```python
from build123d import *

# Parameters (mm, degrees)
SKETCH_1_W          = 51
SKETCH_1_H          = 39
EXTRUDE_1_DEPTH     = 240
SKETCH_2_W          = 41.961119827
SKETCH_2_H          = 6.971123129
EXTRUDE_2_DEPTH     = 35
SKETCH_3_W          = 16.244799638
SKETCH_3_H          = 3.419957818
EXTRUDE_3_DEPTH     = 30
SKETCH_4_W          = 51
SKETCH_4_H          = 4.841751688
EXTRUDE_4_DEPTH     = 10
SKETCH_5_W          = 44.706396848
SKETCH_5_H          = 29.024048215
CUT_EXTRUDE_1_DEPTH = 10
SKETCH_6_W          = 34.715500368
SKETCH_6_H          = 26.036625276
CUT_EXTRUDE_2_DEPTH = 10


with BuildPart() as part:
    # 草图1 → 凸台-拉伸1 (new body)
    with BuildSketch(Plane(origin=(0, 0, 0), x_dir=(1, 0, 0), z_dir=(0, 1, 0))):
        with Locations((25.5, 19.5)):
            Rectangle(SKETCH_1_W, SKETCH_1_H)
    extrude(amount=EXTRUDE_1_DEPTH)

    # 草图2 → 凸台-拉伸2 (add)
    with BuildSketch(Plane(origin=(0, 240, 0), x_dir=(1, 0, 0), z_dir=(0, 1, 0))):
        with Locations((25.724627293, 35.514438435)):
            Rectangle(SKETCH_2_W, SKETCH_2_H)
    extrude(amount=EXTRUDE_2_DEPTH)

    # 草图3 → 凸台-拉伸3 (add)
    with BuildSketch(Plane(origin=(0, 240, 0), x_dir=(1, 0, 0), z_dir=(0, 1, 0))):
        with Locations((21.054054836, 2.926937994)):
            Rectangle(SKETCH_3_W, SKETCH_3_H)
    extrude(amount=EXTRUDE_3_DEPTH)

    # 草图4 → 凸台-拉伸4 (add)
    with BuildSketch(Plane.XZ):
        with Locations((25.5, -36.579124156)):
            Rectangle(SKETCH_4_W, SKETCH_4_H)
    extrude(amount=EXTRUDE_4_DEPTH)

    # 草图5 → 切除-拉伸1 (cut)
    with BuildSketch(Plane.XZ):
        with Locations((25.96812981, -17.773771326)):
            Rectangle(SKETCH_5_W, SKETCH_5_H)
    extrude(amount=-CUT_EXTRUDE_1_DEPTH, mode=Mode.SUBTRACT)

    # 草图6 → 切除-拉伸2 (cut)
    with BuildSketch(Plane.XY.offset(-32.028876871)):
        with Locations((26.608486618, 257.459000656)):
            Rectangle(SKETCH_6_W, SKETCH_6_H)
    extrude(amount=-CUT_EXTRUDE_2_DEPTH, mode=Mode.SUBTRACT)


solid = part.part
```
Here's how the part is built. I have some questions about the finished solid (model axes, mm). A direction names the side the tool comes from. Coordinates: 2 decimals unless noted, no trailing zeros. Write each loop counter-clockwise with the first axis right and the second up, starting at its lowest first coordinate (ties: lowest second). Pieces come first, ordered by that corner, then holes. Notation, with made-up numbers: (-26, 4) - (-17, 4) arc R11 ccw to (-17, 8) - close; hole circle Ø8 at (62.5, 85). An arc over 180 degrees is marked (long way). One line per item, written item: value.
1) Suppose I cut it at B-B on z = -20. Write out the boundary of the cut face in (x, y), and give its area (3 significant figures).
Model answer:
outline: (0, 0) - (3.61, 0) - (3.61, 10) - (48.32, 10) - (48.32, 0) - (51, 0) - (51, 240) - (0, 240) - close
area: 11,800 mm²
2) I'm going to push flat-ended pins straight in: P1, Ø5, axis at y = 2.5, z = -11.5, coming from the -X side; P2, Ø3.5, axis at y = 258, z = -36, coming from the +X side; P3, Ø17.5, axis at x = 34, y = 253, coming from the +Z side; P4, Ø4, axis at y = 253.5, z = -3.5, coming from the -X side. Where does each tip first touch, or does it pass through?
Model answer:
P1: stops at x = 0
P2: stops at x = 46.71
P3: stops at z = -1.22
P4: stops at x = 12.93
3) On a 3-axis mill with a long thin cutter (end or side, diameter ignored), from which of +Z, -Z, +X, -X, +Y, -Y can I reach the whole of each face in a straight line? I mean faces 5 (the flat face through (3.615, 5, -18)), 6 (the flat face through (21, 255, -1.217)), 7 (the flat face through (4.744, 257, -35)), 8 (the flat face through (9.251, 257, -35)), 9 (the flat face through (25, -10, -37)). Say none if no direction works.
Model answer:
face 5: -Y
face 6: +Z, +X, -X, +Y
face 7: +Z, -Z, -X, +Y
face 8: +Z, -Z
face 9: +Z, -Z, +X, -X, -Y
4) I need wall thicknesses on line 1 along X through (y, z) = (8.5, -16); line 2 along Y through (x, z) = (37, -20); line 3 along Y through (x, z) = (13.5, -4). Which ranges of each line are inside material? Lowest first, please.
Model answer:
line 1: x = 0 to 3.61, 48.32 to 51
line 2: y = 10 to 240
line 3: y = 10 to 270
5) We'd pull the mould along Y, two halves only. Please class faces 1 (the flat face through (43.966, 257, -35)), 2 (the flat face through (22, 0, -3)), 3 (the flat face through (26, 270.477, -35)), 4 (the flat face through (25, 118, 0)): pulls with the +Y half, pulls with the -Y half, needs draft (parallel to the pull), parting line crosses it, or undercut.
Model answer:
face 1: undercut
face 2: pulls with the -Y half
face 3: undercut
face 4: needs draft
6) Suppose I cut it at C-C on x = 38. Write out the boundary of the cut face in (y, z), and give its area (3 significant figures).
Model answer:
outline: (-10, -39) - (244.44, -39) - (244.44, -32.03) - (240, -32.03) - (240, 0) - (0, 0) - (0, -3.26) - (10, -3.26) - (10, -32.29) - (0, -32.29) - (0, -34.16) - (-10, -34.16) - close; (270.48, -39) - (275, -39) - (275, -32.03) - (270.48, -32.03) - close
area: 9,180 mm²
7) Suppose I cut it at A-A on x = 21. Write out the boundary of the cut face in (y, z).
Model answer:
outline: (-10, -39) - (244.44, -39) - (244.44, -32.03) - (240, -32.03) - (240, -4.64) - (270, -4.64) - (270, -1.22) - (240, -1.22) - (240, 0) - (0, 0) - (0, -3.26) - (10, -3.26) - (10, -32.29) - (0, -32.29) - (0, -34.16) - (-10, -34.16) - close; (270.48, -39) - (275, -39) - (275, -32.03) - (270.48, -32.03) - close
